from build123d import *

# Parameters (mm, degrees)
SKETCH_1_W          = 280
SKETCH_1_H          = 20
EXTRUDE_1_DEPTH     = 40
SKETCH_2_R          = 3.5
CUT_EXTRUDE_1_DEPTH = 30


with BuildPart() as part:
    # 스케치1 → 보스-돌출1 (new body)
    with BuildSketch(Plane.XY):
        Rectangle(SKETCH_1_W, SKETCH_1_H)
    extrude(amount=EXTRUDE_1_DEPTH)

    # 스케치2 → 컷-돌출1 (cut)
    with BuildSketch(Plane.XZ.offset(10)):
        with Locations(Location((-134.5, 25.5, 0), (0, 0, 270))):
            Circle(SKETCH_2_R)
        with Locations(Location((-134.5, 14.5, 0), (0, 0, 270))):
            Circle(SKETCH_2_R)
        with Locations(Location((134.5, 24.5, 0), (0, 0, 270))):
            Circle(SKETCH_2_R)
        with Locations(Location((134.5, 13.5, 0), (0, 0, 270))):
            Circle(SKETCH_2_R)
    extrude(amount=-CUT_EXTRUDE_1_DEPTH, mode=Mode.SUBTRACT)


solid = part.part
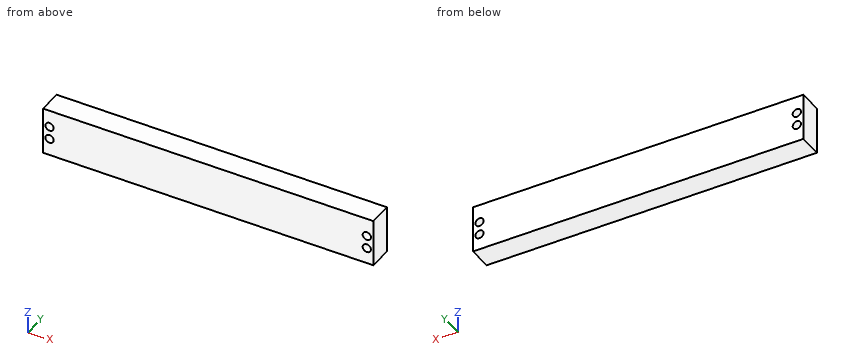
Geometry check sheet. Reference: the model listing, model coordinates, mm. Round coordinates to 2 decimals unless told otherwise and drop trailing zeros. Loops run counter-clockwise (first coordinate to the right, second up) from the corner with the lowest first, then second, coordinate; pieces in that order, holes last. Notation, with made-up numbers: (33.5, 42) - (75.5, 42) arc R34 cw to (75.5, 79) - close; hole circle Ø10 at (88.5, 1.5). An arc over 180 degrees is marked (long way). Answer as CSV lines item,"result".
(1) Material ranges on line 1 along Z through (x, y) = (134.5, -0.75); line 2 along X through (y, z) = (-3.5, 11.5); line 3 along X through (y, z) = (-3, 14.5), recorded low to high.
Output values:
line 1,"z = 0 to 10, 17 to 21, 28 to 40"
line 2,"x = -140 to -136.3, -132.7 to 131.63, 137.37 to 140"
line 3,"x = -140 to -138, -131 to 131.15, 137.85 to 140"
(2) Cross-section at B-B, the plane z = 13.5. Enter the section's corners in (x, y), and give its area (3 significant figures).
Output values:
outline,"(-140, -10) - (-137.85, -10) - (-137.85, 10) - (-140, 10) - close; (-131.15, -10) - (131, -10) - (131, 10) - (-131.15, 10) - close; (138, -10) - (140, -10) - (140, 10) - (138, 10) - close"
area,"5,330 mm²"
(3) Cross-section at A-A, the plane x = -134.5. Enter the section's corners in (y, z).
Output values:
outline,"(-10, 0) - (10, 0) - (10, 11) - (-10, 11) - close; (-10, 18) - (10, 18) - (10, 22) - (-10, 22) - close; (-10, 29) - (10, 29) - (10, 40) - (-10, 40) - close"
